The drawing under review shows one solid part. Ordinate dimensions are in mm from its lowest x, y, z. A direction names the side the tool comes from. Give positions to 0.01 mm unless a question says otherwise; leave off trailing zeros. Order: outer loops, then holes, each group sorted by start corner. A loop starts at its lowest first (then second) coordinate and runs counter-clockwise, first axis right, second up. Notation, with made-up numbers: (17, 32.25) -> (36, 32.25) arc R16 ccw to (36, 56.25) -> close; hole circle Ø8 at (70, 47). An arc over 180 degrees is marked (long way). One line per item, written item: value.
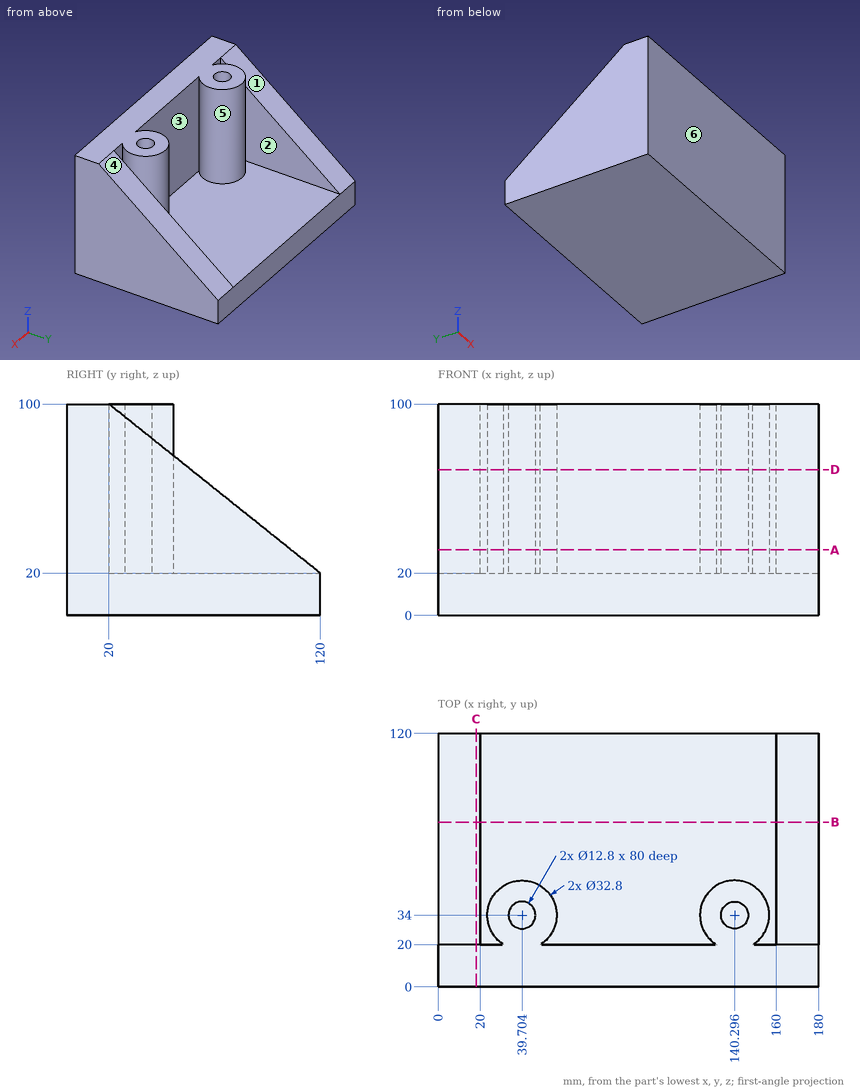
Item 1: To check wall thickness, follow line 1 along X through (y, z) = (48, 47.5); line 2 along X through (y, z) = (57, 26.5); line 3 along X through (y, z) = (44, 27). State the ranges of each line that lie inside material, in increasing order. Write a range as from..to.
Returned:
line 1: 0..20, 31.16..48.25, 131.75..148.84, 160..180
line 2: 0..20, 160..180
line 3: 0..20, 26.71..52.7, 127.3..153.29, 160..180
Item 2: Draft analysis for pull direction Y (two halves, no side actions). For the marked faces 4, 5 and 6, state which applies: pulls with the +Y half, pulls with the -Y half, needs draft (parallel to the pull), parting line crosses it, or undercut.
Returned:
face 4: pulls with the +Y half
face 5: undercut
face 6: pulls with the -Y half
Item 3: Clearance check with flat-ended pins moving along their axes: P1, Ø1, axis at x = 68.5, z = 19.5, coming from the -Y side; P2, Ø3.5, axis at x = 154.5, z = 72, coming from the +Y side; P3, Ø10, axis at x = 76, z = 38.5, coming from the +Y side; P4, Ø10, axis at x = 39.704, y = 34, coming from the +Z side. State where each tip first meets the part, or that it passes through.
Returned:
P1: y = 0
P2: y = 44.67
P3: y = 20
P4: z = 20
Item 4: Add section D-D on z = 69. Give the boundary of the cut face in (x, y), plus the area to 3 significant figures.
Returned:
outline: (0, 0) -> (180, 0) -> (180, 58.75) -> (160, 58.75) -> (160, 20) -> (148.84, 20) arc R16.4 ccw (long way) to (131.75, 20) -> (48.25, 20) arc R16.4 ccw (long way) to (31.16, 20) -> (20, 20) -> (20, 58.75) -> (0, 58.75) -> close; hole circle Ø12.8 at (39.7, 34); hole circle Ø12.8 at (140.3, 34)
area: 6,530 mm²
Item 5: Add section A-A on z = 31. Give the boundary of the cut face in (x, y), plus the area to 3 significant figures.
Returned:
outline: (0, 0) -> (180, 0) -> (180, 106.25) -> (160, 106.25) -> (160, 20) -> (148.84, 20) arc R16.4 ccw (long way) to (131.75, 20) -> (48.25, 20) arc R16.4 ccw (long way) to (31.16, 20) -> (20, 20) -> (20, 106.25) -> (0, 106.25) -> close; hole circle Ø12.8 at (39.7, 34); hole circle Ø12.8 at (140.3, 34)
area: 8,430 mm²
Item 6: Add section C-C on x = 18. Give the boundary of the cut face in (y, z).
Returned:
outline: (0, 0) -> (120, 0) -> (120, 20) -> (20, 100) -> (0, 100) -> close
Item 7: Machinability: for the marked faces 1, 2 and 3, which of the approach directions +Z, -Z, +X, -X, +Y, -Y give a long, thin tool a straight path to every point of the face, cutting with its end or side? Answer none if there is none.
Returned:
face 1: +Z, -X, +Y
face 2: +Z, +Y
face 3: +Z
Item 8: Add section B-B on y = 78. Give the boundary of the cut face in (x, z), plus the area to 3 significant figures.
Returned:
outline: (0, 0) -> (180, 0) -> (180, 53.6) -> (160, 53.6) -> (160, 20) -> (20, 20) -> (20, 53.6) -> (0, 53.6) -> close
area: 4,940 mm²
